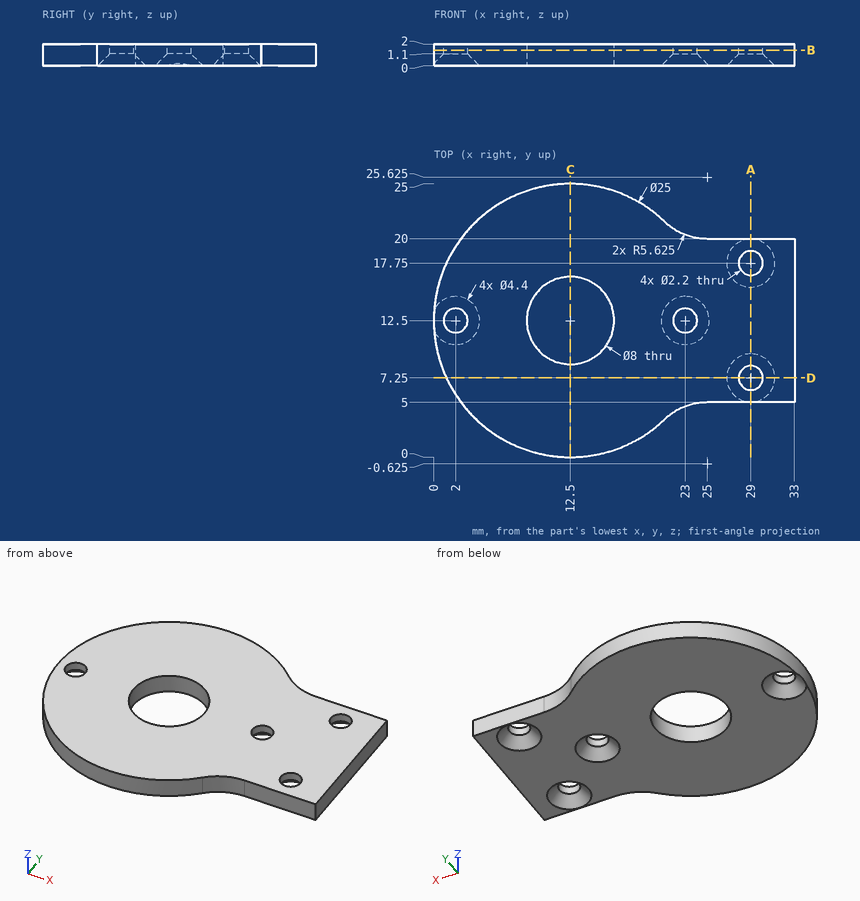
Job drawing, mm, ordinate dimensions from the low corner. One solid piece. Round coordinates to 2 decimals unless told otherwise and drop trailing zeros. Order: outer loops, then holes, each group sorted by start corner. A loop starts at its lowest first (then second) coordinate and runs counter-clockwise, first axis right, second up. Notation, with made-up numbers: (31, -1) -> (55, -1) arc R15 cw to (55, 22) -> close; hole circle Ø11 at (37, 81.5). An arc over 180 degrees is marked (long way). Write item = value, one per line.
(1) Cut at A-A (x = 29). Write the cut outline in (y, z).
Answers follow:
outline = (5, 0) -> (5.05, 0) -> (6.15, 1.1) -> (6.15, 2) -> (5, 2) -> close; (8.35, 1.1) -> (9.45, 0) -> (15.55, 0) -> (16.65, 1.1) -> (16.65, 2) -> (8.35, 2) -> close; (18.85, 1.1) -> (19.95, 0) -> (20, 0) -> (20, 2) -> (18.85, 2) -> close
(2) Cut at B-B (z = 1.45). Write the cut outline in (x, y) (3 decimals), plus the area to 3 significant figures.
Answers follow:
outline = (21.121, 3.448) arc R5.625 cw to (25, 5) -> (33, 5) -> (33, 20) -> (25, 20) arc R5.625 cw to (21.121, 21.552) arc R12.5 ccw (long way) to start; hole circle Ø2.2 at (2, 12.5); hole circle Ø8 at (12.5, 12.5); hole circle Ø2.2 at (23, 12.5); hole circle Ø2.2 at (29, 7.25); hole circle Ø2.2 at (29, 17.75)
area = 559 mm²
(3) Flat gauge pins, fed straight in: P1, Ø0.6, axis at x = 27.5, z = 1, coming from the -Y side; P2, Ø0.6, axis at x = 27.5, z = 1, coming from the +Y side; P3, Ø1, axis at x = 20.5, z = 1, coming from the -Y side. Where does each tip first touch, or does it go through?
Answers follow:
P1 = 5
P2 = 20
P3 = 2.5
(4) Drill centre lines: L1, parallel to Y at x = 12.5, z = 1.25; L2, parallel to Y at x = 31.5, z = 0.4; L3, parallel to Y at x = 27.5, z = 0.15. Where is each one in solid material? Low to high.
Answers follow:
L1 = 0 to 8.5, 16.5 to 25
L2 = 5 to 20
L3 = 5 to 5.85, 8.65 to 16.35, 19.15 to 20
(5) Cut at C-C (x = 12.5). Write the cut outline in (y, z).
Answers follow:
outline = (0, 0) -> (8.5, 0) -> (8.5, 2) -> (0, 2) -> close; (16.5, 0) -> (25, 0) -> (25, 2) -> (16.5, 2) -> close
(6) Cut at D-D (y = 7.25). Write the cut outline in (x, z).
Answers follow:
outline = (1.16, 0) -> (26.8, 0) -> (27.9, 1.1) -> (27.9, 2) -> (1.16, 2) -> close; (30.1, 1.1) -> (31.2, 0) -> (33, 0) -> (33, 2) -> (30.1, 2) -> close
